Build history of the part. All positions in model axes, mm. A direction names the side the tool comes from. Round coordinates to 2 decimals unless told otherwise and drop trailing zeros. Loops run counter-clockwise (first coordinate to the right, second up) from the corner with the lowest first, then second, coordinate; pieces in that order, holes last. Notation, with made-up numbers: M 14,-21 L 66,-21 A17 ccw 66,-16 Z; hole C 84,30.25 d3. An arc over 180 degrees is marked long. One line per item, written item: value.
Autodesk Fusion 360 part; units mm, degrees
sketch "Boceto1" plane through (0, 0, 0) normal (0, 1, 0) x (1, 0, 0)
  line L0 (-45, 25) -> (-4, 25)
  line L1 (-45, 25) -> (-45, -44)
  line L2 (-45, -44) -> (-4, -44)
  line L3 (-4, -44) -> (-4, 25)
  dimension "d1" = 41
  dimension "d2" = 69
extrude "Extruir1" add sketch "Boceto1" along normal blind 31
sketch "Boceto2" plane through (0, 31, 0) normal (0, 1, 0) x (-1, 0, 0)
  line L0 (45, -25) -> (45, 44)
  line L1 (45, 44) -> (4, 44)
  line L2 (4, 44) -> (4, -25)
  line L3 (4, -25) -> (45, -25)
  line L4 (42, 41) -> (42, 31.833)
  line L5 (42, 41) -> (7, 41)
  line L6 (7, 41) -> (7, 6)
  line L7 (7, 6) -> (42, 6)
  line L8 (42, 6) -> (42, 31.833)
  dimension "d7" = 35
  dimension "d8" = 35
extrude "Extruir2" cut sketch "Boceto2" against normal blind 15 contours L4 L5 L6 L7 L8
sketch "Boceto3" plane through (0, 0, 44) normal (0, 0, 1) x (1, 0, 0)
  line L0 (-45, 0) -> (-4, 0)
  line L1 (-4, 0) -> (-4, 31)
  line L2 (-4, 31) -> (-45, 31)
  line L3 (-45, 31) -> (-45, 0)
  line L4 (-45, 0) -> (-45, 13)
  line L5 (-45, 13) -> (-4, 13)
  line L6 (-4, 13) -> (-4, 0)
  dimension "d11" = 13
extrude "Extruir3" cut sketch "Boceto3" against normal blind 38 contours L0 L1 L3 L4 L5 L6
sketch "Boceto4" plane through (0, 31, 0) normal (0, 1, 0) x (-1, 0, 0)
  line L0 (7, 6) -> (7, 41)
  line L1 (7, 41) -> (42, 41)
  line L2 (42, 41) -> (42, 6)
  line L3 (42, 6) -> (7, 6)
  line L4 (45, -25) -> (45, 44)
  line L5 (45, 44) -> (4, 44)
  line L6 (4, 44) -> (4, -25)
  line L7 (4, -25) -> (45, -25)
  line L8 (31, -25) -> (18, -25)
  line L9 (31, -25) -> (31, 3)
  line L10 (31, 3) -> (18, 3)
  line L11 (18, 3) -> (18, -25)
  dimension "d14" = 14
  dimension "d15" = 13
  dimension "d16" = 28
extrude "Extruir4" cut sketch "Boceto4" against normal blind 28 contours L7 L8 L9 L10 L11
sketch "Boceto5" plane through (-45, 0, 0) normal (-1, 0, 0) x (0, 0, 1)
  line L0 (6, 0) -> (6, 13)
  line L1 (6, 13) -> (44, 13)
  line L2 (44, 13) -> (44, 31)
  line L3 (44, 31) -> (-25, 31)
  line L4 (-25, 31) -> (-25, 0)
  line L5 (-25, 0) -> (6, 0)
  line L6 (-25, 31) -> (-10, 31)
  line L7 (-10, 31) -> (-10, 13)
  line L8 (-10, 13) -> (-25, 13)
  line L9 (-25, 13) -> (-25, 31)
  dimension "d19" = 15
  dimension "d20" = 18
extrude "Extruir5" cut sketch "Boceto5" against normal blind 50 contours L3 L4 L6 L7 L8 L9
sketch "Boceto6" plane through (0, 0, 6) normal (0, 0, 1) x (1, 0, 0)
  line L0 (-45, 0) -> (-4, 0)
  line L1 (-4, 0) -> (-4, 13)
  line L2 (-4, 13) -> (-45, 13)
  line L3 (-45, 13) -> (-45, 0)
  line L4 (-31, 13) -> (-18, 13)
  line L5 (-18, 13) -> (-18, 3)
  line L6 (-18, 3) -> (-31, 3)
  line L7 (-31, 3) -> (-31, 13)
  dimension "d23" = 14
  dimension "d24" = 13
  dimension "d25" = 10
extrude "Extruir6" cut sketch "Boceto6" against normal blind 30 contours L2 L4 L5 L6 L7
sketch "Boceto7" plane through (0, 0, 3) normal (0, 0, -1) x (-1, 0, 0)
  line L0 (18, 13) -> (31, 13)
  line L1 (31, 13) -> (31, 31)
  line L2 (31, 31) -> (18, 31)
  line L3 (18, 31) -> (18, 13)
  line L4 (18, 13) -> (31, 13)
  line L5 (31, 13) -> (31, 22.5)
  line L6 (31, 22.5) -> (18, 22.5)
  line L7 (18, 22.5) -> (18, 13)
  dimension "d28" = 9.5
extrude "Extruir7" add sketch "Boceto7" along normal blind 4.5 contours L0 L1 L3 L4 L5 L6 L7
sketch "Boceto8" plane through (0, 13, 0) normal (0, -1, 0) x (1, 0, 0)
  line L0 (-4, 44) -> (-45, 44)
  line L1 (-45, 44) -> (-45, 6)
  line L2 (-45, 6) -> (-31, 6)
  line L3 (-31, 6) -> (-31, -1.5)
  line L4 (-31, -1.5) -> (-18, -1.5)
  line L5 (-18, -1.5) -> (-18, 6)
  line L6 (-18, 6) -> (-4, 6)
  line L7 (-4, 6) -> (-4, 44)
  line L8 (-45, 44) -> (-35, 44)
  line L9 (-35, 44) -> (-35, 34)
  line L10 (-35, 34) -> (-45, 34)
  line L11 (-45, 34) -> (-45, 44)
  line L12 (-4, 44) -> (-14, 44)
  line L13 (-14, 44) -> (-14, 34)
  line L14 (-14, 34) -> (-4, 34)
  line L15 (-4, 34) -> (-4, 44)
extrude "Extruir8" add sketch "Boceto8" along normal blind 13 contours L0 L7 L12 L13 L14 L15 | L0 L1 L8 L9 L10 L11
sketch "Boceto9" plane through (0, 0, 0) normal (0, -1, 0) x (1, 0, 0)
  line L0 (-45, 34) -> (-35, 34)
  line L1 (-35, 34) -> (-35, 44)
  line L2 (-35, 44) -> (-45, 44)
  line L3 (-45, 44) -> (-45, 34)
  line L4 (-40, 34) -> (-40, 39)
  line L5 (-40, 39) -> (-35, 39)
  line L6 (-35, 34) -> (-40, 34)
  line L7 (-14, 34) -> (-9, 34)
  line L8 (-14, 34) -> (-14, 39)
  line L9 (-14, 39) -> (-9, 39)
  line L10 (-9, 39) -> (-9, 34)
extrude "Extruir9" cut sketch "Boceto9" against normal blind 13 contours L0 L1 L4 L5 L6 | L7 L8 L9 L10
sketch "Boceto10" plane through (0, 22.5, 0) normal (0, 1, 0) x (-1, 0, 0)
  line L0 (31, 3) -> (18, 3)
  line L1 (18, 3) -> (18, -1.5)
  line L2 (18, -1.5) -> (31, -1.5)
  line L3 (31, -1.5) -> (31, 3)
  circle A0 centre (24.5, 0.75) radius 0.5
  dimension "d35" = 1
extrude "Extruir10" cut sketch "Boceto10" against normal blind 4 contours A0
extrude "Extruir11" add 1 faces at (-22.3333, 3, -14.6667) along direction (0, 1, 0) blind 3
extrude "Extruir12" cut 1 faces at (-22.3333, 6, -14.6667) along direction (0, -1, 0) blind 3
extrude "Extruir13" cut 1 faces at (-29, 22.5, 0.75) along direction (0, -1, 0) blind 3
extrude "Extruir14" cut 1 faces at (-24.1479, 18.5, 0.7889) along direction (0, -1, 0) blind 3
Item 1: Wall check: line 1 along Z through (x, y) = (-24.5, 16.8); line 2 along X through (y, z) = (27.5, -2.5); line 3 along Z through (x, y) = (-27, 23). Give the ranges that are in metal, low to high.
Check values:
line 1: z = -1.5 to 0.25, 1.25 to 6, 41 to 44
line 2: x = -45 to -31, -18 to -4
line 3: z = 3 to 6, 41 to 44
Item 2: Pull direction Z, two halves, no side cores. Call faces 6 (the face through (-11, 22, -10)), 7 (the face through (-25, 31, 5)), 8 (the face through (-12, 6, 39)): pulls with the +Z half, pulls with the -Z half, needs draft (parallel to the pull), parting line crosses it, or undercut.
Check values:
face 6: pulls with the -Z half
face 7: needs draft
face 8: undercut
Item 3: Slice it at C-C, the plane x = -10.5. Give the cut face in (y, z), and give its area (3 significant figures).
Check values:
outline: M 0,-25 L 13,-25 L 13,-10 L 31,-10 L 31,6 L 16,6 L 16,41 L 31,41 L 31,44 L 0,44 L 0,39 L 13,39 L 13,6 L 0,6 Z
area: 915 mm2
Item 4: Slice it at A-A, the plane y = 5. Give the cut face in (x, z), and give its area (3 significant figures).
Check values:
outline: M -45,-25 L -31,-25 L -31,6 L -45,6 Z; M -45,34 L -40,34 L -40,39 L -35,39 L -35,44 L -45,44 Z; M -18,-25 L -4,-25 L -4,6 L -18,6 Z; M -14,39 L -9,39 L -9,34 L -4,34 L -4,44 L -14,44 Z
area: 1,020 mm2
Item 5: Drop flat-ended pins along their axis: P1, Ø7, axis at x = -36, z = -14, coming from the +Y side; P2, Ø16.5, axis at x = -24.5, y = 27, coming from the -Z side; P3, Ø2, axis at x = -30, z = 35.5, coming from the +Y side. Give the stop position or say it passes through.
Check values:
P1: stops at y = 13
P2: stops at z = -10
P3: stops at y = 16
Item 6: Slice it at B-B, the plane y = 23.5. Give the cut face in (x, z).
Check values:
outline: M -45,-10 L -31,-10 L -31,3 L -18,3 L -18,-10 L -4,-10 L -4,44 L -45,44 Z; hole M -42,6 L -7,6 L -7,41 L -42,41 Z
Item 7: Slice it at D-D, the plane z = 14. Give the cut face in (x, y), and give its area (3 significant figures).
Check values:
outline: M -45,13 L -4,13 L -4,31 L -7,31 L -7,16 L -42,16 L -42,31 L -45,31 Z
area: 213 mm2
Item 8: Which spindle directions (+Z, -Z, +X, -X, +Y, -Y) get a long thin tool onto all of the face, cutting with end or side? Do faces 1 (the face through (-31, 14, -6)), 2 (the face through (-25, 24, 41)), 3 (the face through (-11, 13, -17)), 4 (the face through (-25, 25, 3)), 5 (the face through (-24, 2, 6)). Say none if no direction does.
Check values:
face 1: -Z
face 2: +Y
face 3: -Z, +X, -X, +Y
face 4: -Z, +Y
face 5: +X, -X, -Y
